Part model, mm, in its own coordinate system. Face numbers are marked on the shaded views. A direction names the side the tool comes from. Round coordinates to 2 decimals unless told otherwise and drop trailing zeros. Write each loop counter-clockwise with the first axis right and the second up, starting at its lowest first coordinate (ties: lowest second). Pieces come first, ordered by that corner, then holes. Notation, with made-up numbers: M -21,17 L -17,17 A27 cw -17,55 Z; hole C 71,-19 d3. An arc over 180 degrees is marked long. Answer as a JSON object with one key per item and string values. Group by question number.
1. Which spindle directions (+Z, -Z, +X, -X, +Y, -Y) get a long thin tool onto all of the face, cutting with end or side? Do the marked faces 4 and 5. Say none if no direction does.
2. Two-plate mould, pull along Y, no slides. Class the marked faces 1, 2 and 3: +Y half, -Y half, draft (parallel to the pull), parting line (faces both ways), or undercut.
3. Drill centre lines: line 1 (Y direction, x = 11.43, z = 9); line 2 (Y direction, x = -9.5, z = 34); line 3 (Z direction, x = -8, y = 35). Where is each one in solid material? Low to high. Write a range as from..to.
4. Band-saw the part on D-D, the plane z = 13.5. Write the cut outline in (x, y), plus the area to 3 significant figures.
5. Band-saw the part on B-B, the plane y = 12.7. Write the cut outline in (x, z), plus the area to 3 significant figures.
6. Band-saw the part on A-A, the plane z = 19.05. Write the cut outline in (x, y), plus the area to 3 significant figures.
7. Drop a flat-ended pin along its axis: pin 1 (19 mm diameter, centred on y = -11.5, z = 19, fed in from -X). Give the stop position or say it passes through.
8. Band-saw the part on C-C, the plane x = 11.43. Write the cut outline in (y, z).
from build123d import *

# Parameters (mm, degrees)
SKETCH1_W           = 38.1
SKETCH1_H           = 76.2
BOSS_EXTRUDE1_DEPTH = 38.1
SKETCH2_W           = 22.86
SKETCH2_H           = 63.5
CUT_EXTRUDE1_DEPTH  = 38.1
SKETCH3_R           = 5.1181
SKETCH3_R_2         = 1.8034
CUT_EXTRUDE2_DEPTH  = 38.1
SKETCH4_R           = 1.6256
SKETCH4_R_2         = 1.8034
CUT_EXTRUDE3_DEPTH  = 76.2


with BuildPart() as part:
    # Sketch1 → Boss-Extrude1 (new body)
    with BuildSketch(Plane.XY):
        Rectangle(SKETCH1_W, SKETCH1_H)
    extrude(amount=BOSS_EXTRUDE1_DEPTH)

    # Sketch2 → Cut-Extrude1 (cut)
    with BuildSketch(Plane(origin=(0, 0, 0), x_dir=(-1, 0, 0), z_dir=(0, 0, -1))):
        with Locations((7.62, 0)):
            Rectangle(SKETCH2_W, SKETCH2_H)
    extrude(amount=-CUT_EXTRUDE1_DEPTH, mode=Mode.SUBTRACT)

    # Sketch3 → Cut-Extrude2 (cut)
    with BuildSketch(Plane(origin=(0, 0, 0), x_dir=(-1, 0, 0), z_dir=(0, 0, -1))):
        with Locations((-11.43, 0)):
            Circle(SKETCH3_R)
        with Locations((-11.43, -12.7)):
            Circle(SKETCH3_R_2)
        with Locations((-11.43, 12.7)):
            Circle(SKETCH3_R_2)
    extrude(amount=-CUT_EXTRUDE2_DEPTH, mode=Mode.SUBTRACT)

    # Sketch4 → Cut-Extrude3 (cut)
    with BuildSketch(Plane(origin=(0, -38.1, 0), x_dir=(-1, 0, 0), z_dir=(0, -1, 0))):
        with Locations(Location((8.89, -6.35, 0), (0, 0, 90))):
            Circle(SKETCH4_R)
        with Locations(Location((8.89, -19.05, 0), (0, 0, 90))):
            Circle(SKETCH4_R_2)
        with Locations(Location((8.89, -31.75, 0), (0, 0, 90))):
            Circle(SKETCH4_R)
    extrude(amount=-CUT_EXTRUDE3_DEPTH, mode=Mode.SUBTRACT)


solid = part.part
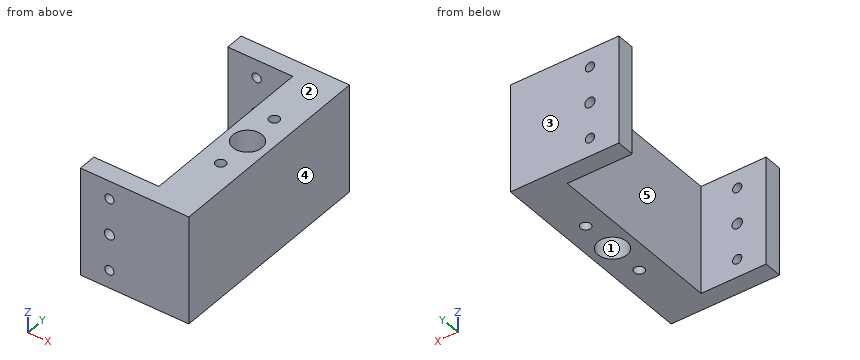
Worked answers:
{
 "1": {"face 4": "+Z, -Z, +X, +Y, -Y", "face 5": "+Z, -Z, -X"},
 "2": {"face 1": "undercut", "face 2": "draft", "face 3": "+Y half"},
 "3": {"line 1": "y = -38.1..-14.5, -10.9..-5.12, 5.12..10.9, 14.5..38.1", "line 2": "y = -38.1..-31.75, 31.75..38.1", "line 3": "z = 0..4.99, 7.71..17.48, 20.62..30.39, 33.11..38.1"},
 "4": {"outline": "M -19.05,-38.1 L 19.05,-38.1 L 19.05,38.1 L -19.05,38.1 L -19.05,31.75 L 3.81,31.75 L 3.81,-31.75 L -19.05,-31.75 Z; hole C 11.43,0 d10.24; hole C 11.43,-12.7 d3.61; hole C 11.43,12.7 d3.61", "area": "1,350 mm^2"},
 "5": {"outline": "M 3.81,0 L 9.63,0 L 9.63,38.1 L 3.81,38.1 Z; M 13.23,0 L 19.05,0 L 19.05,38.1 L 13.23,38.1 Z", "area": "443 mm^2"},
 "6": {"outline": "M -19.05,-38.1 L -10.69,-38.1 L -10.69,-31.75 L -19.05,-31.75 Z; M -19.05,31.75 L -10.69,31.75 L -10.69,38.1 L -19.05,38.1 Z; M -7.09,-38.1 L 19.05,-38.1 L 19.05,38.1 L -7.09,38.1 L -7.09,31.75 L 3.81,31.75 L 3.81,-31.75 L -7.09,-31.75 Z; hole C 11.43,0 d10.24; hole C 11.43,-12.7 d3.61; hole C 11.43,12.7 d3.61", "area": "1,300 mm^2"},
 "7": {"pin 1": "stops at x = 3.81"},
 "8": {"outline": "M -38.1,0 L -14.5,0 L -14.5,38.1 L -38.1,38.1 Z; M -10.9,0 L -5.12,0 L -5.12,38.1 L -10.9,38.1 Z; M 5.12,0 L 10.9,0 L 10.9,38.1 L 5.12,38.1 Z; M 14.5,0 L 38.1,0 L 38.1,38.1 L 14.5,38.1 Z"}
}
